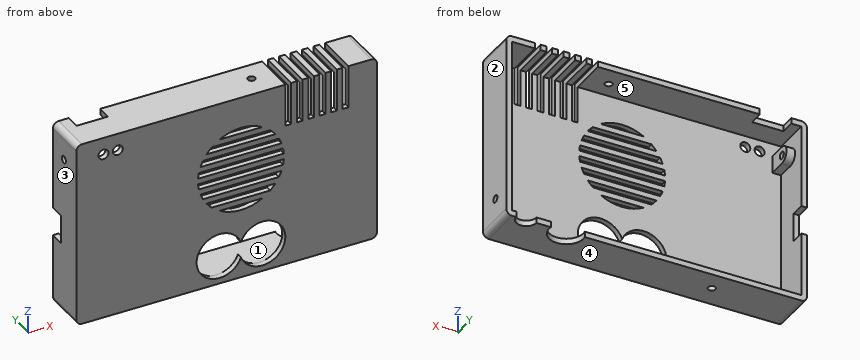
from build123d import *

# Parameters (mm, degrees)
SKETCH_1_W           = 105
SKETCH_1_H           = 65.5
EXTRUDE_1_DEPTH      = 15
SHELL_1_T            = -2
FILLET_1_R           = 2
SKETCH_2_W           = 10
SKETCH_2_H           = 5
CUT_EXTRUDE_1_DEPTH  = 14
SKETCH_3_W           = 11
SKETCH_3_H           = 5
CUT_EXTRUDE_2_DEPTH  = 14
SKETCH_5_W           = 2
SKETCH_5_H           = 17.663494354
CUT_EXTRUDE_3_DEPTH  = 15
SKETCH_6_R           = 3.5
SKETCH_6_R_2         = 6
CUT_EXTRUDE_4_DEPTH  = 15
CUT_EXTRUDE_5_DEPTH  = 15
CUT_EXTRUDE_6_DEPTH  = 15
SKETCH_9_R           = 1.75
CUT_EXTRUDE_7_DEPTH  = 15
SKETCH_10_R          = 1.3
CUT_EXTRUDE_8_DEPTH  = 15
SKETCH_12_R          = 1.3
CUT_EXTRUDE_9_DEPTH  = 15
EXTRUDE_3_DEPTH      = 3
SKETCH_16_R          = 1.3
CUT_EXTRUDE_11_DEPTH = 8
SKETCH_17_R          = 1.3
CUT_EXTRUDE_12_DEPTH = 39
SKETCH_18_R          = 1.3
CUT_EXTRUDE_13_DEPTH = 39


with BuildPart() as part:
    # 草图1 → 凸台-拉伸1 (new body)
    with BuildSketch(Plane(origin=(0, 0, 0), x_dir=(1, 0, 0), z_dir=(0, 1, 0))):
        Rectangle(SKETCH_1_W, SKETCH_1_H)
    extrude(amount=EXTRUDE_1_DEPTH)

    # 抽壳1
    shell_1_openings = [part.faces().sort_by_distance(p)[0] for p in [
        (0, 15, 0),
    ]]
    offset(amount=SHELL_1_T, openings=shell_1_openings, kind=Kind.INTERSECTION)

    # 圆角1
    fillet_1_edges = [part.edges().sort_by_distance(p)[0] for p in [
        (-52.5, 7.5, -32.75),
        (52.5, 7.5, -32.75),
        (52.5, 7.5, 32.75),
        (-52.5, 7.5, 32.75),
    ]]
    fillet(fillet_1_edges, radius=FILLET_1_R)

    # 草图2 → 切除-拉伸1 (cut)
    with BuildSketch(Plane.ZY.offset(52.5)):
        with Locations((-3.25, 12.5)):
            Rectangle(SKETCH_2_W, SKETCH_2_H)
    extrude(amount=-CUT_EXTRUDE_1_DEPTH, mode=Mode.SUBTRACT)

    # 草图3 → 切除-拉伸2 (cut)
    with BuildSketch(Plane.XY.offset(32.75)):
        with Locations((-41.5, 12.5)):
            Rectangle(SKETCH_3_W, SKETCH_3_H)
    extrude(amount=-CUT_EXTRUDE_2_DEPTH, mode=Mode.SUBTRACT)

    # 草图5 → 切除-拉伸3 (cut)
    with BuildSketch(Plane.XY.offset(32.75)):
        with Locations((41.5, 6.168252823)):
            Rectangle(SKETCH_5_W, SKETCH_5_H)
        with Locations((37.5, 6.168252823)):
            Rectangle(SKETCH_5_W, SKETCH_5_H)
        with Locations((33.5, 6.168252823)):
            Rectangle(SKETCH_5_W, SKETCH_5_H)
        with Locations((29.5, 6.168252823)):
            Rectangle(SKETCH_5_W, SKETCH_5_H)
        with Locations((25.5, 6.168252823)):
            Rectangle(SKETCH_5_W, SKETCH_5_H)
        with Locations((21.5, 6.168252823)):
            Rectangle(SKETCH_5_W, SKETCH_5_H)
    extrude(amount=-CUT_EXTRUDE_3_DEPTH, mode=Mode.SUBTRACT)

    # 草图6 → 切除-拉伸4 (cut)
    with BuildSketch(Plane(origin=(0, 0, -32.75), x_dir=(-1, 0, 0), z_dir=(0, 0, -1))):
        with Locations((-45.5, 15)):
            Circle(SKETCH_6_R)
        with Locations((-31, 14)):
            Circle(SKETCH_6_R_2)
    extrude(amount=-CUT_EXTRUDE_4_DEPTH, mode=Mode.SUBTRACT)

    # 草图7 → 切除-拉伸5 (cut)
    with BuildSketch(Plane(origin=(0, 2, 0), x_dir=(1, 0, 0), z_dir=(0, 1, 0))):
        with BuildLine():
            ThreePointArc((5, 19.966117819), (20.5, 22.75), (5, 25.533882181))
            ThreePointArc((5, 25.533882181), (-10.5, 22.75), (5, 19.966117819))
        make_face()
    extrude(amount=-CUT_EXTRUDE_5_DEPTH, mode=Mode.SUBTRACT)

    # 草图8 → 切除-拉伸6 (cut)
    with BuildSketch(Plane.XZ):
        with BuildLine():
            Line((-2.483314774, 19.75), (12.483314774, 19.75))
            ThreePointArc((12.483314774, 19.75), (5, 21.75), (-2.483314774, 19.75))
        make_face()
        with BuildLine():
            Line((-5.198039027, 17.75), (15.198039027, 17.75))
            ThreePointArc((15.198039027, 17.75), (16.143977484, 16.790506254), (17, 15.75))
            Line((17, 15.75), (-7, 15.75))
            ThreePointArc((-7, 15.75), (-6.143977484, 16.790506254), (-5.198039027, 17.75))
        make_face()
        with BuildLine():
            Line((-8.266499161, 13.75), (18.266499161, 13.75))
            ThreePointArc((18.266499161, 13.75), (18.740753807, 12.765952527), (19.142135624, 11.75))
            Line((19.142135624, 11.75), (-9.142135624, 11.75))
            ThreePointArc((-9.142135624, 11.75), (-8.740753807, 12.765952527), (-8.266499161, 13.75))
        make_face()
        with BuildLine():
            Line((-9.696938457, 9.75), (19.696938457, 9.75))
            ThreePointArc((19.696938457, 9.75), (19.865457163, 8.754540676), (19.966629547, 7.75))
            Line((19.966629547, 7.75), (-9.966629547, 7.75))
            ThreePointArc((-9.966629547, 7.75), (-9.865457163, 8.754540676), (-9.696938457, 9.75))
        make_face()
        with BuildLine():
            Line((-9.966629547, 5.75), (19.966629547, 5.75))
            ThreePointArc((19.966629547, 5.75), (19.865457163, 4.745459324), (19.696938457, 3.75))
            Line((19.696938457, 3.75), (-9.696938457, 3.75))
            ThreePointArc((-9.696938457, 3.75), (-9.865457163, 4.745459324), (-9.966629547, 5.75))
        make_face()
        with BuildLine():
            Line((-9.142135624, 1.75), (19.142135624, 1.75))
            ThreePointArc((19.142135624, 1.75), (18.740753807, 0.734047473), (18.266499161, -0.25))
            Line((18.266499161, -0.25), (-8.266499161, -0.25))
            ThreePointArc((-8.266499161, -0.25), (-8.740753807, 0.734047473), (-9.142135624, 1.75))
        make_face()
        with BuildLine():
            Line((-7, -2.25), (17, -2.25))
            ThreePointArc((17, -2.25), (16.143977484, -3.290506254), (15.198039027, -4.25))
            Line((15.198039027, -4.25), (-5.198039027, -4.25))
            ThreePointArc((-5.198039027, -4.25), (-6.143977484, -3.290506254), (-7, -2.25))
        make_face()
        with BuildLine():
            Line((-2.483314774, -6.25), (12.483314774, -6.25))
            ThreePointArc((12.483314774, -6.25), (5, -8.25), (-2.483314774, -6.25))
        make_face()
    extrude(amount=-CUT_EXTRUDE_6_DEPTH, mode=Mode.SUBTRACT)

    # 草图9 → 切除-拉伸7 (cut)
    with BuildSketch(Plane(origin=(0, 2, 0), x_dir=(1, 0, 0), z_dir=(0, 1, 0))):
        with Locations(Location((-43, -26.75, 0), (0, 0, 270))):
            Circle(SKETCH_9_R)
        with Locations(Location((-38, -26.75, 0), (0, 0, 270))):
            Circle(SKETCH_9_R)
    extrude(amount=-CUT_EXTRUDE_7_DEPTH, mode=Mode.SUBTRACT)

    # 草图10 → 切除-拉伸8 (cut)
    with BuildSketch(Plane.ZY.offset(52.5)):
        with Locations((23.25, 8)):
            Circle(SKETCH_10_R)
    extrude(amount=-CUT_EXTRUDE_8_DEPTH, mode=Mode.SUBTRACT)

    # 草图12 → 切除-拉伸9 (cut)
    with BuildSketch(Plane(origin=(52.5, 0, 0), x_dir=(0, 0, -1), z_dir=(1, 0, 0))):
        with Locations((23.25, 8)):
            Circle(SKETCH_12_R)
    extrude(amount=-CUT_EXTRUDE_9_DEPTH, mode=Mode.SUBTRACT)

    # 草图13 → 凸台-拉伸3 (add)
    with BuildSketch(Plane(origin=(-50.5, 0, 0), x_dir=(0, 0, -1), z_dir=(1, 0, 0))):
        with BuildLine():
            Line((-26.25, 8), (-26.25, 2))
            Line((-26.25, 2), (-20.25, 2))
            Line((-20.25, 2), (-20.25, 8))
            ThreePointArc((-20.25, 8), (-23.25, 11), (-26.25, 8))
        make_face()
    extrude(amount=EXTRUDE_3_DEPTH)

    # 草图16 → 切除-拉伸11 (cut)
    with BuildSketch(Plane.ZY.offset(50.5)):
        with Locations((23.25, 8)):
            Circle(SKETCH_16_R)
    extrude(amount=-CUT_EXTRUDE_11_DEPTH, mode=Mode.SUBTRACT)

    # 草图17 → 切除-拉伸12 (cut)
    with BuildSketch(Plane.XY.offset(32.75)):
        with Locations((13, 8)):
            Circle(SKETCH_17_R)
    extrude(amount=-CUT_EXTRUDE_12_DEPTH, mode=Mode.SUBTRACT)

    # 草图18 → 切除-拉伸13 (cut)
    with BuildSketch(Plane(origin=(0, 0, -32.75), x_dir=(-1, 0, 0), z_dir=(0, 0, -1))):
        with Locations((23, 8)):
            Circle(SKETCH_18_R)
    extrude(amount=-CUT_EXTRUDE_13_DEPTH, mode=Mode.SUBTRACT)


solid = part.part
For this review, take the finished solid that the model builds, in its own axes (mm). Face numbers are marked on the shaded views. A direction names the side the tool comes from. Round coordinates to 2 decimals unless told otherwise and drop trailing zeros. Order: outer loops, then holes, each group sorted by start corner. A loop starts at its lowest first (then second) coordinate and runs counter-clockwise, first axis right, second up. Notation, with made-up numbers: M 73.5,8.5 L 100.5,8.5 A19 ccw 100.5,18.5 Z; hole C 41.25,37 d9. An arc over 180 degrees is marked long. Use a Markdown table: item, result. Add a question column.
Item 1: Add section A-A, the plane x = -23. Give the boundary of the cut face in (y, z), then the cut area to 3 significant figures.
Item 2: Add section C-C, the plane x = -38. Give the boundary of the cut face in (y, z), then the cut area to 3 significant figures.
Item 3: To check wall thickness, follow line 1 along X through (y, z) = (5.25, 12); line 2 along Z through (x, y) = (10.5, 10.25); line 3 along X through (y, z) = (3, 23). State the ranges of each line that lie inside material, in increasing order.
Item 4: Tool access review of the marked faces 1 and 2: name each direction out of +Z, -Z, +X, -X, +Y, -Y from which nothing blocks a thin tool from reaching the whole face with its end or side.
Item 5: Add section D-D, the plane z = 23.25. State how many separate pieces and enclosed holes the cut face has, then the cut area to 3 significant figures.
Item 6: Add section B-B, the plane z = -29. Give the boundary of the cut face in (x, y).
Item 7: Insertion check: pin 1 (0.6 mm diameter, centred on x = -39.5, z = 31.5, fed in from +Y); pin 2 (6 mm diameter, centred on x = -6, z = 25, fed in from +Y); pin 3 (2 mm diameter, centred on x = 25, y = 1, fed in from +Z); pin 4 (0.6 mm diameter, centred on x = 41.5, y = 1, fed in from +Z). Each pin has a flat end and moves straight along its axis. Give the tip position at first contact, or say it passes through.
Item 8: Mouldability with a two-part tool opening along Z and no side actions: class the marked faces 3, 4 and 5 as released by +Z, released by -Z, zero draft, split by the parting line, or undercut.
Geometry results:
| question | item | result |
|---|---|---|
| 1 | outline | M 0,-32.75 L 6.7,-32.75 L 6.7,-30.75 L 2,-30.75 L 2,30.75 L 15,30.75 L 15,32.75 L 0,32.75 Z; M 9.3,-32.75 L 15,-32.75 L 15,-30.75 L 9.3,-30.75 Z |
| 1 | area | 178 mm² |
| 2 | outline | M 0,-32.75 L 15,-32.75 L 15,-30.75 L 2,-30.75 L 2,25 L 0,25 Z; M 0,28.5 L 2,28.5 L 2,30.75 L 10,30.75 L 10,32.75 L 0,32.75 Z |
| 2 | area | 166 mm² |
| 3 | line 1 | x = -52.5 to -50.5, 50.5 to 52.5 |
| 3 | line 2 | z = -32.75 to -30.75, 30.75 to 32.75 |
| 3 | line 3 | x = -52.5 to -47.5, 50.5 to 52.5 |
| 4 | face 1 | +Y |
| 4 | face 2 | +Z, -Z, +X, +Y, -Y |
| 5 | separate pieces | 8 |
| 5 | enclosed holes | 0 |
| 5 | area | 252 mm² |
| 6 | outline | M -52.5,0 L -7.49,0 L -7.49,2 L -50.5,2 L -50.5,15 L -52.5,15 Z; M 2.49,0 L 7.51,0 L 7.51,2 L 2.49,2 Z; M 17.49,0 L 52.5,0 L 52.5,15 L 50.5,15 L 50.5,2 L 17.49,2 Z |
| 7 | pin 1 | stops at y = 10 |
| 7 | pin 2 | stops at y = 2 |
| 7 | pin 3 | stops at z = 32.75 |
| 7 | pin 4 | stops at z = 17.75 |
| 8 | face 3 | zero draft |
| 8 | face 4 | released by -Z |
| 8 | face 5 | undercut |
